from build123d import *

# Parameters (mm, degrees)
F1_DEPTH = 24
F2_T     = -2
F3_R     = 8.25
F4_DEPTH = 2
F5_R     = 2
F5_R_2   = 0.7
F6_DEPTH = 13
F7_W     = 13
F7_H     = 11
F8_DEPTH = 2


with BuildPart() as f1:
    # F0 (on Top) → F1 (new body)
    with BuildSketch(Plane.XY):
        with BuildLine():
            ThreePointArc((42.5, 29.5), (41.6213203436, 31.6213203436), (39.5, 32.5))
            Line((39.5, 32.5), (-39.5, 32.5))
            ThreePointArc((-39.5, 32.5), (-41.6213203436, 31.6213203436), (-42.5, 29.5))
            Line((-42.5, 29.5), (-42.5, -29.5))
            ThreePointArc((-42.5, -29.5), (-41.6213203436, -31.6213203436), (-39.5, -32.5))
            Line((-39.5, -32.5), (39.5, -32.5))
            ThreePointArc((39.5, -32.5), (41.6213203436, -31.6213203436), (42.5, -29.5))
            Line((42.5, -29.5), (42.5, 29.5))
        make_face()
    extrude(amount=F1_DEPTH)

    # F2
    f2_openings = [f1.faces().sort_by_distance(p)[0] for p in [
        (0, 0, 24),
    ]]
    offset(amount=F2_T, openings=f2_openings)

    # F3 (on face) → F4 (cut, through all)
    with BuildSketch(Plane.XY.offset(2)):
        with Locations((19.05, 18.25)):
            Circle(F3_R)
    extrude(amount=-F4_DEPTH, mode=Mode.SUBTRACT)

    # F5 (on face) → F6 (join)
    with BuildSketch(Plane.XY.offset(2)):
        with Locations((-37.5, 27.5)):
            Circle(F5_R)
        with Locations((-37.5, 27.5)):
            Circle(F5_R_2, mode=Mode.SUBTRACT)
        with Locations((37.5, 27.5)):
            Circle(F5_R)
        with Locations((37.5, 27.5)):
            Circle(F5_R_2, mode=Mode.SUBTRACT)
        with Locations((37.5, -27.5)):
            Circle(F5_R)
        with Locations((37.5, -27.5)):
            Circle(F5_R_2, mode=Mode.SUBTRACT)
        with Locations((-37.5, -27.5)):
            Circle(F5_R)
        with Locations((-37.5, -27.5)):
            Circle(F5_R_2, mode=Mode.SUBTRACT)
    extrude(amount=F6_DEPTH)

    # F7 (on face) → F8 (cut, through all)
    with BuildSketch(Plane.XZ.offset(32.5)):
        with Locations((10, 10.5)):
            Rectangle(F7_W, F7_H)
        with Locations((-25, 10.5)):
            Rectangle(F7_W, F7_H)
    extrude(amount=-F8_DEPTH, mode=Mode.SUBTRACT)


solid = f1.part
Build history of the part. All positions in model axes, mm. A direction names the side the tool comes from. Round coordinates to 2 decimals unless told otherwise and drop trailing zeros. Write each loop counter-clockwise with the first axis right and the second up, starting at its lowest first coordinate (ties: lowest second). Pieces come first, ordered by that corner, then holes. Notation, with made-up numbers: M -13.5,-16 L 5.5,-16 A23 ccw 5.5,22 Z; hole C 80.5,10.25 d3. An arc over 180 degrees is marked long. Use CSV: the item, a comma, the result in double quotes.
1. Saw through at D-D (z = 17.25). Give the cut face in (x, y).
Reply:
outline,"M -42.5,-29.5 A3 ccw -39.5,-32.5 L 39.5,-32.5 A3 ccw 42.5,-29.5 L 42.5,29.5 A3 ccw 39.5,32.5 L -39.5,32.5 A3 ccw -42.5,29.5 Z; hole M -40.5,-29.5 A1 ccw -39.5,-30.5 L 39.5,-30.5 A1 ccw 40.5,-29.5 L 40.5,29.5 A1 ccw 39.5,30.5 L -39.5,30.5 A1 ccw -40.5,29.5 Z"
2. Saw through at C-C (x = 19.05). Give the cut face in (y, z), plus the area to 3 significant figures.
Reply:
outline,"M -32.5,0 L 10,0 L 10,2 L -30.5,2 L -30.5,24 L -32.5,24 Z; M 26.5,0 L 32.5,0 L 32.5,24 L 30.5,24 L 30.5,2 L 26.5,2 Z"
area,"185 mm²"
3. Saw through at B-B (z = 8.5). State how many separate pieces and enclosed holes the cut face has, plus the area to 3 significant figures.
Reply:
separate pieces,"6"
enclosed holes,"4"
area,"569 mm²"
4. Flat gauge pins, fed straight in: pin 1 (1.2 mm diameter, centred on x = 38.5, y = 28.5, fed in from +Z); pin 2 (1.3 mm diameter, centred on x = -37.5, y = 27.5, fed in from +Z). Where does each tip first touch, or does it go through?
Reply:
pin 1,"stops at z = 15"
pin 2,"stops at z = 2"
5. Two-plate mould, pull along Z, no slides. Class faces 4 (the face through (-25, -32, 5)), 5 (the face through (-1, 0, 2)), 6 (the face through (-1, -32.5, 12)), 7 (the face through (-25, -32, 16)): +Z half, -Z half, draft (parallel to the pull), parting line (faces both ways), or undercut.
Reply:
face 4,"undercut"
face 5,"+Z half"
face 6,"draft"
face 7,"undercut"
6. Wall check: probe 1 along Y at (x, z) = (-37.5, 10); probe 2 along X at (y, z) = (13, 3); probe 3 along Y at (x, z) = (-19, 4). Give the ranges that are in metal, low to high. Write a range as from..to.
Reply:
probe 1,"y = -32.5..-30.5, -29.5..-28.2, -26.8..-25.5, 25.5..26.8, 28.2..29.5, 30.5..32.5"
probe 2,"x = -42.5..-40.5, 40.5..42.5"
probe 3,"y = -32.5..-30.5, 30.5..32.5"
7. Saw through at A-A (y = 18.25). Give the cut face in (x, z), plus the area to 3 significant figures.
Reply:
outline,"M -42.5,0 L 10.8,0 L 10.8,2 L -40.5,2 L -40.5,24 L -42.5,24 Z; M 27.3,0 L 42.5,0 L 42.5,24 L 40.5,24 L 40.5,2 L 27.3,2 Z"
area,"225 mm²"
8. Tool access for faces 1 (the face through (40.5, 0, 13)), 2 (the face through (-42.5, 0, 12)), 3 (the face through (10, -32, 5)): list every direction of +Z, -Z, +X, -X, +Y, -Y with a clear straight run to the whole face (end or side of a thin tool).
Reply:
face 1,"+Z"
face 2,"+Z, -Z, -X, +Y, -Y"
face 3,"-Y"
